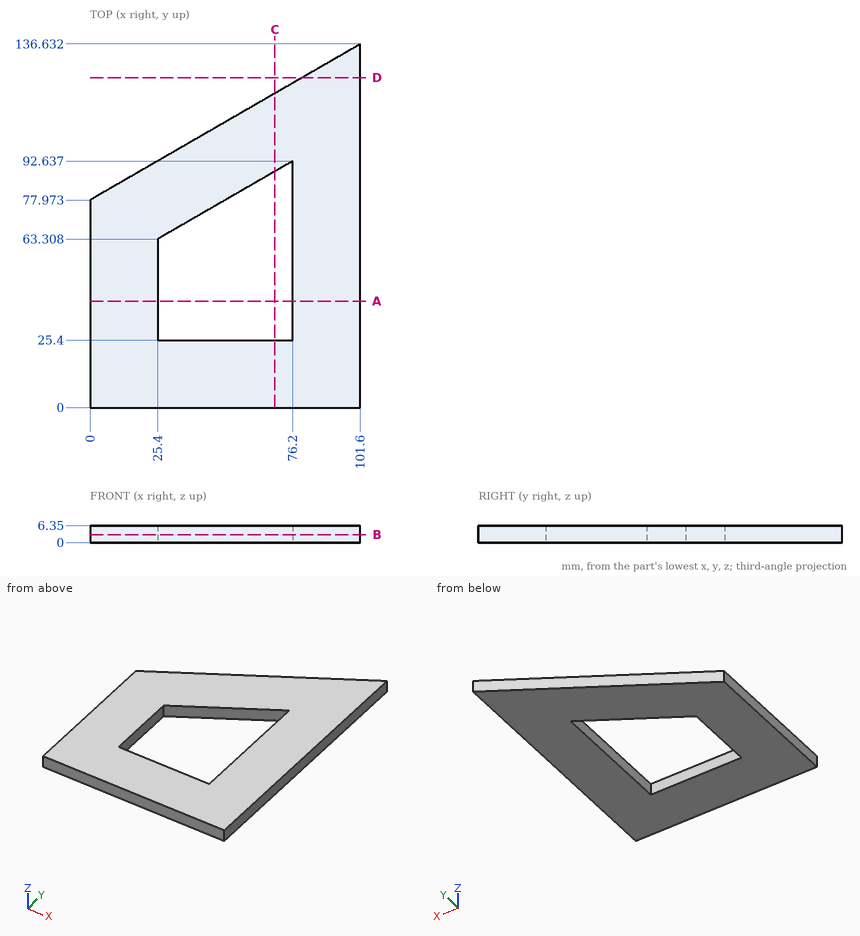
Could you check a few things on this drawing? It's one solid part, dimensions in mm from its lowest x, y, z. Give positions to 0.01 mm unless a question says otherwise; leave off trailing zeros. Write each loop counter-clockwise with the first axis right and the second up, starting at its lowest first coordinate (ties: lowest second). Pieces come first, ordered by that corner, then holes. Notation, with made-up numbers: (22, 50.5) -> (46, 50.5) arc R28 ccw to (46, 87.5) -> close; hole circle Ø3 at (18.25, 18.25). An arc over 180 degrees is marked (long way). Write item = value, one per line.
(1) Suppose I cut it at B-B on z = 3. Write out the boundary of the cut face in (x, y).
Worked out:
outline = (0, 0) -> (101.6, 0) -> (101.6, 136.63) -> (0, 77.97) -> close; hole (25.4, 25.4) -> (76.2, 25.4) -> (76.2, 92.64) -> (25.4, 63.31) -> close
(2) I need wall thicknesses on probe 1 along X at (y, z) = (33.5, 1); probe 2 along Y at (x, z) = (56.5, 5.25) (1 decimal); probe 3 along Y at (x, z) = (53, 2.75). Which ranges of each line are inside material? Lowest first, please. Write a range as from..to.
Worked out:
probe_1 = 0..25.4, 76.2..101.6
probe_2 = 0..25.4, 81.3..110.6
probe_3 = 0..25.4, 79.24..108.57
(3) I'm going to push flat-ended pins straight in: P1, Ø3, axis at x = 86, z = 1, coming from the +Y side; P2, Ø3, axis at x = 41.5, z = 4.5, coming from the +Y side. Where does each tip first touch, or does it pass through?
Worked out:
P1 = 128.49
P2 = 102.8
(4) Suppose I cut it at A-A on y = 40. Write out the boundary of the cut face in (x, z).
Worked out:
outline = (0, 0) -> (25.4, 0) -> (25.4, 6.35) -> (0, 6.35) -> close; (76.2, 0) -> (101.6, 0) -> (101.6, 6.35) -> (76.2, 6.35) -> close
(5) Suppose I cut it at C-C on x = 69.5. Write out the boundary of the cut face in (y, z).
Worked out:
outline = (0, 0) -> (25.4, 0) -> (25.4, 6.35) -> (0, 6.35) -> close; (88.77, 0) -> (118.1, 0) -> (118.1, 6.35) -> (88.77, 6.35) -> close
(6) Suppose I cut it at D-D on y = 124. Write out the boundary of the cut face in (x, z).
Worked out:
outline = (79.72, 0) -> (101.6, 0) -> (101.6, 6.35) -> (79.72, 6.35) -> close
